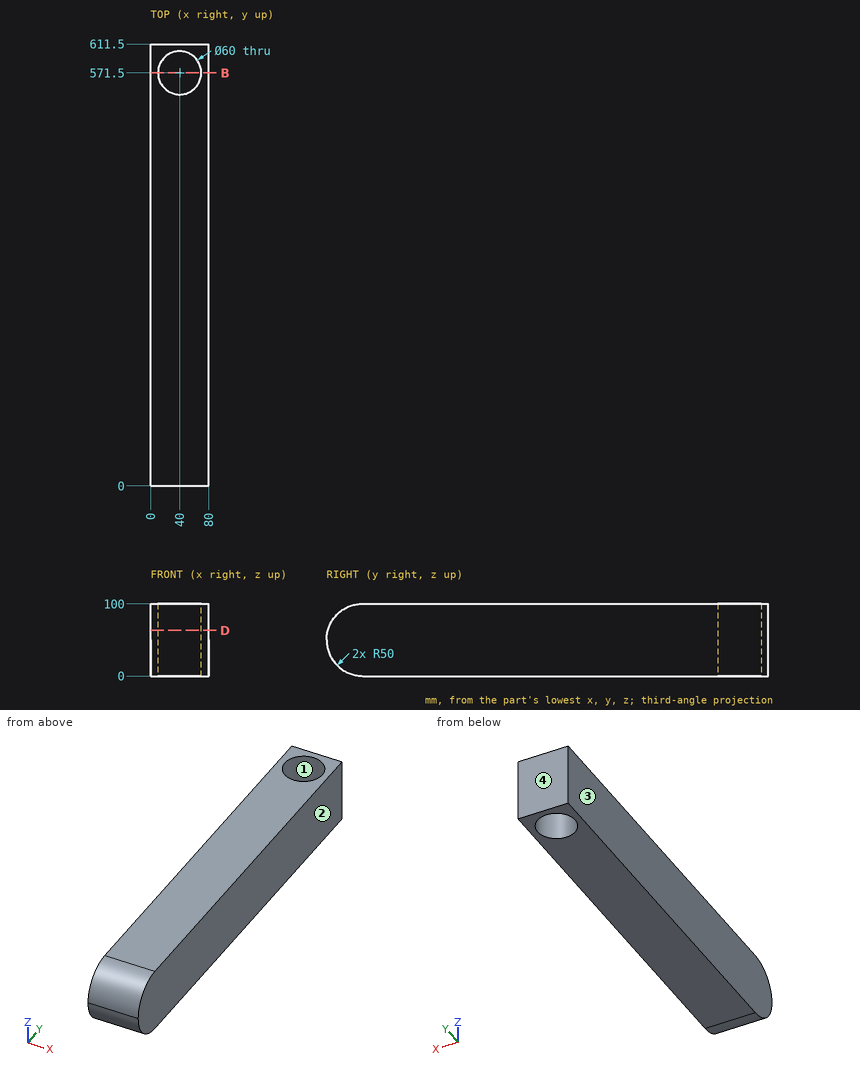
For this review, use the dimensioned drawing (mm, ordinates from the lowest corner) and the shaded views. Round coordinates to 2 decimals unless told otherwise and drop trailing zeros. Loops run counter-clockwise (first coordinate to the right, second up) from the corner with the lowest first, then second, coordinate; pieces in that order, holes last. Notation, with made-up numbers: (-8.75, 22.25) -> (8.25, 22.25) arc R18 cw to (8.25, 30.25) -> close; hole circle Ø4 at (69.5, 5.25). An arc over 180 degrees is marked (long way). Write item = value, one per line. Start each with the question number.
Item 1: Take a section at D-D on z = 63. Give the boundary of the cut face in (x, y).
Item 2: Mouldability with a two-part tool opening along X and no side actions: class the marked faces 1, 2, 3 and 4 as released by +X, released by -X, zero draft, split by the parting line, or undercut.
Item 3: To check wall thickness, follow L1, parallel to X at y = 571, z = 65; L2, parallel to Y at x = 40, z = 47.5; L3, parallel to Y at x = 40, z = 21.5. State the ranges of each line that lie inside material, in increasing order.
Item 4: Insertion check: pin 1 (2 mm diameter, centred on x = 67.5, z = 54, fed in from -Y); pin 2 (1.5 mm diameter, centred on x = 36.5, z = 36.5, fed in from -Y). Each pin has a flat end and moves straight along its axis. Give the tip position at first contact, or say it passes through.
Item 5: Take a section at B-B on y = 571.5. Give the boundary of the cut face in (x, z).
Result:
q1.outline = (0, 1.72) -> (80, 1.72) -> (80, 611.5) -> (0, 611.5) -> close; hole circle Ø60 at (40, 571.5)
q2.face_1 = undercut
q2.face_2 = released by +X
q2.face_3 = released by -X
q2.face_4 = zero draft
q3.L1 = 0 to 10, 70 to 80
q3.L2 = 0.06 to 541.5, 601.5 to 611.5
q3.L3 = 8.92 to 541.5, 601.5 to 611.5
q4.pin_1 = 0.09
q4.pin_2 = 1.65
q5.outline = (0, 0) -> (10, 0) -> (10, 100) -> (0, 100) -> close; (70, 0) -> (80, 0) -> (80, 100) -> (70, 100) -> close
